Work out the finished part from the listing and answer in its coordinate system (mm). Round coordinates to 2 decimals unless told otherwise and drop trailing zeros. Loops run counter-clockwise (first coordinate to the right, second up) from the corner with the lowest first, then second, coordinate; pieces in that order, holes last.
```python
from build123d import *

# Parameters (mm, degrees)
F0_W     = 101.6
F0_H     = 101.6
F0_W_2   = 91.44
F0_H_2   = 91.44
F1_DEPTH = 101.6
F2_W     = 91.44
F2_H     = 91.44
F3_DEPTH = 101.6
F4_W     = 91.44
F4_H     = 91.44
F5_DEPTH = 101.6
F6_W     = 91.44
F6_H     = 91.44
F7_DEPTH = 25.4


with BuildPart() as f1:
    # F0 (on Top) → F1 (new body)
    with BuildSketch(Plane.XY):
        Rectangle(F0_W, F0_H)
        Rectangle(F0_W_2, F0_H_2, mode=Mode.SUBTRACT)
        Rectangle(F0_W_2, F0_H_2)
    extrude(amount=F1_DEPTH)

    # F2 (on face) → F3 (cut)
    with BuildSketch(Plane.YZ.offset(50.8)):
        with Locations((0, 50.8)):
            Rectangle(F2_W, F2_H)
    extrude(amount=-F3_DEPTH, mode=Mode.SUBTRACT)

    # F4 (on face) → F5 (cut)
    with BuildSketch(Plane.XZ.offset(50.8)):
        with Locations((0, 50.8)):
            Rectangle(F4_W, F4_H)
    extrude(amount=-F5_DEPTH, mode=Mode.SUBTRACT)

    # F6 (on face) → F7 (cut)
    with BuildSketch(Plane.XY.offset(101.6)):
        Rectangle(F6_W, F6_H)
    extrude(amount=-F7_DEPTH, mode=Mode.SUBTRACT)


solid = f1.part
```
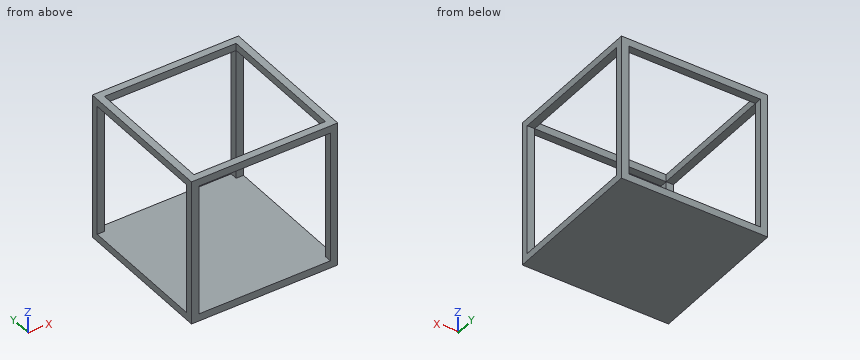
1. Given pin 1 (5 mm diameter, centred on x = 13, y = 2, fed in from +Z), flat-ended and moving along its own axis, determine where the tip first touches the part or whether it passes through.
Answer key:
pin 1: stops at z = 5.08
2. Consider probe 1 along Z at (x, y) = (8.5, 22). Determine where the line is inside the solid, lowest interval first.
Answer key:
probe 1: z = 0 to 5.08
3. Find section A-A (y = -11.5). Write down the section's boundary in (x, z).
Answer key:
outline: (-50.8, 0) - (50.8, 0) - (50.8, 5.08) - (-50.8, 5.08) - close; (-50.8, 96.52) - (-45.72, 96.52) - (-45.72, 101.6) - (-50.8, 101.6) - close; (45.72, 96.52) - (50.8, 96.52) - (50.8, 101.6) - (45.72, 101.6) - close
4. Find section C-C (z = 87). Write down the section's boundary in (x, y).
Answer key:
outline: (-50.8, -50.8) - (-45.72, -50.8) - (-45.72, -45.72) - (-50.8, -45.72) - close; (-50.8, 45.72) - (-45.72, 45.72) - (-45.72, 50.8) - (-50.8, 50.8) - close; (45.72, -50.8) - (50.8, -50.8) - (50.8, -45.72) - (45.72, -45.72) - close; (45.72, 45.72) - (50.8, 45.72) - (50.8, 50.8) - (45.72, 50.8) - close
